Input: part model. Units: mm. Frame: model coordinates. Give positions to 0.01 mm unless a question says otherwise; leave off trailing zeros. Loops run counter-clockwise (first coordinate to the right, second up) from the corner with the lowest first, then second, coordinate; pieces in that order, holes last. Notation, with made-up numbers: (17.25, 19.5) - (24.25, 19.5) arc R30 cw to (24.25, 54.5) - close; hole circle Ø1 at (24, 60.5). An arc over 180 degrees is marked (long way). Answer as a JSON object with one key per item and string values.
Autodesk Inventor part; units mm, degrees
ref_plane "YZ Plane" through (0, 0, 0) normal (1, 0, 0) x (0, 1, 0)
ref_plane "XZ Plane" through (0, 0, 0) normal (0, 1, 0) x (-1, 0, 0)
ref_plane "XY Plane" through (0, 0, 0) normal (0, 0, 1) x (1, 0, 0)
sketch "Sketch1" plane through (0, 0, 0) normal (0, 1, 0) x (-1, 0, 0)
  line L0 (200, 0) -> (185, 0)
  line L1 (200, 0) -> (215, 0) construction
  line L2 (185, 0) -> (185, -30)
  line L3 (185, -30) -> (115, -30)
  line L4 (115, -30) -> (115, 0)
  line L5 (200, -140) -> (185, -140)
  line L6 (200, -140) -> (215, -140) construction
  line L7 (185, -140) -> (185, -110)
  line L8 (185, -110) -> (115, -110)
  line L9 (115, -110) -> (115, -140)
  line L10 (200, 0) -> (197, 0)
  line L11 (197, 0) -> (197, -140)
  line L12 (197, 0) -> (337, 0) construction
  line L13 (200, 0) -> (200, -20)
  line L14 (200, -20) -> (200, -40)
  line L15 (200, -40) -> (200, -60)
  line L16 (200, -60) -> (200, -80)
  line L17 (200, -80) -> (200, -100)
  line L18 (200, -100) -> (200, -120)
  line L19 (200, -120) -> (200, -140)
  line L20 (200, -20) -> (197, -20)
  line L21 (200, -40) -> (197, -40)
  line L22 (200, -60) -> (197, -60)
  line L23 (200, -80) -> (197, -80)
  line L24 (200, -100) -> (197, -100)
  line L25 (200, -120) -> (197, -120)
  line L26 (100, 0) -> (100, -140)
  line L27 (100, -140) -> (200, -140)
  line L28 (100, 0) -> (200, 0)
  line L29 (0, 0) -> (15, 0)
  line L30 (0, 0) -> (-15, 0) construction
  line L31 (15, 0) -> (15, -30)
  line L32 (15, -30) -> (85, -30)
  line L33 (85, -30) -> (85, 0)
  line L34 (85, -110) -> (85, -140)
  line L35 (15, -140) -> (15, -110)
  line L36 (15, -110) -> (85, -110)
  line L37 (0, -140) -> (15, -140)
  line L38 (0, -140) -> (-15, -140) construction
  line L39 (0, 0) -> (3, 0)
  line L40 (3, 0) -> (3, -140)
  line L41 (3, 0) -> (-137, 0) construction
  line L42 (0, 0) -> (0, -20)
  line L43 (0, -20) -> (0, -40)
  line L44 (0, -40) -> (0, -60)
  line L45 (0, -60) -> (0, -80)
  line L46 (0, -80) -> (0, -100)
  line L47 (0, -100) -> (0, -120)
  line L48 (0, -120) -> (0, -140)
  line L49 (0, -20) -> (3, -20)
  line L50 (0, -40) -> (3, -40)
  line L51 (0, -60) -> (3, -60)
  line L52 (0, -80) -> (3, -80)
  line L53 (0, -100) -> (3, -100)
  line L54 (0, -120) -> (3, -120)
  line L55 (100, -140) -> (0, -140)
  line L56 (100, 0) -> (0, 0)
  dimension "d2" = 15
  dimension "d3" = 180
  dimension "d4" = 30
  dimension "d5" = 70
  dimension "d6" = 90
  dimension "d12" = 3
  dimension "d13" = 140
  dimension "d14" = 90
  dimension "d15" = 20
  dimension "d16" = 20
  dimension "d17" = 20
  dimension "d18" = 20
  dimension "d19" = 20
  dimension "d20" = 20
  dimension "d21" = 20
extrude "Extrusion1" add sketch "Sketch1" along normal blind 3 contours L13 L20 L11 L0 | L11 L5 L7 L8 L9 L27 L26 L28 L4 L3 L2 L0 | L15 L22 L11 L21 | L26 L55 L34 L36 L35 L37 L40 L29 L31 L32 L33 L56 | L17 L24 L11 L23 | L19 L5 L11 L25 | L40 L49 L42 L29 | L37 L48 L54 L40 | L40 L51 L44 L50 | L53 L46 L52 L40
properties part number "onderkant"
Item 1: Contact query for flat-ended pins moving along their axis: P1, Ø1.5, axis at x = -151, y = 2, coming from the +Z side; P2, Ø1.5, axis at y = 1.5, z = -110, coming from the +X side. Output: stop coordinate, or through.
Geometry check:
{"P1": "stops at z = -30", "P2": "stops at x = -3"}
Item 2: Cut plane C-C (x = -79). Return loops of the section in (y, z).
Geometry check:
{"outline": "(0, -110) - (3, -110) - (3, -30) - (0, -30) - close"}
Item 3: Material intervals for line 1 (X direction, y = 1.15, z = -12.5); line 2 (X direction, y = 2.1, z = -69.5); line 3 (Z direction, x = -18, y = 1.95), sorted ascending. Write a range as [from, to].
Geometry check:
{"line 1": "x = [-200, -185], [-115, -85], [-15, 0]", "line 2": "x = [-197, -3]", "line 3": "z = [-110, -30]"}
Item 4: Cut plane A-A (z = -123). Return loops of the section in (x, y), then the cut area to 3 significant figures.
Geometry check:
{"outline": "(-200, 0) - (-185, 0) - (-185, 3) - (-200, 3) - close; (-115, 0) - (-85, 0) - (-85, 3) - (-115, 3) - close; (-15, 0) - (0, 0) - (0, 3) - (-15, 3) - close", "area": "180 mm2"}
Item 5: Cut plane B-B (z = -28). Return loops of the section in (x, y).
Geometry check:
{"outline": "(-197, 0) - (-185, 0) - (-185, 3) - (-197, 3) - close; (-115, 0) - (-85, 0) - (-85, 3) - (-115, 3) - close; (-15, 0) - (-3, 0) - (-3, 3) - (-15, 3) - close"}
